Autodesk Inventor part; units mm, degrees
ref_plane "YZ Plane" through (0, 0, 0) normal (1, 0, 0) x (0, 1, 0)
ref_plane "XZ Plane" through (0, 0, 0) normal (0, 1, 0) x (-1, 0, 0)
ref_plane "XY Plane" through (0, 0, 0) normal (0, 0, 1) x (1, 0, 0)
sketch "Sketch1" plane through (0, 0, 0) normal (0, 1, 0) x (-1, 0, 0)
  line L0 (65, 0) -> (65, -110)
  line L1 (65, -110) -> (0, -110)
  line L2 (0, -110) -> (0, 0)
  line L3 (65, 0) -> (65, -34.9842)
  line L4 (65, 0) -> (50.25, 0)
  line L5 (50.25, 0) -> (50.25, -30.5)
  line L6 (0, 0) -> (14.75, 0)
  line L7 (14.75, 0) -> (14.75, -30.5)
  line L8 (50.25, -30.5) -> (14.75, -30.5)
  line L9 (0, 0) -> (14.75, 0)
  line L10 (50.25, 0) -> (65, 0)
  dimension "d0" = 65
  dimension "d1" = 110
  dimension "d2" = 14.75
  dimension "d3" = 30.5
  dimension "d4" = 14.75
  dimension "d5" = 30.5
extrude "Extrusion1" add sketch "Sketch1" along normal blind 18.5
sketch "Sketch2" plane through (0, 18.5, 0) normal (0, 1, 0) x (1, 0, 0)
  line L0 (0, 110) -> (-65, 110)
  line L1 (-65, 110) -> (-65, 0)
  line L2 (-14.75, 0) -> (0, 0)
  line L3 (-65, 0) -> (0, 0)
  line L4 (0, 0) -> (0, 110)
  line L5 (-65, 110) -> (-65, 0)
  line L6 (0, 110) -> (-65, 110)
extrude "Extrusion2" add sketch "Sketch2" along normal blind 10
sketch "Sketch3" plane through (0, 0, 0) normal (0, -1, 0) x (1, 0, 0)
  line L0 (0, 0) -> (0, -110)
  line L1 (0, -110) -> (-65, -110)
  line L2 (0, 0) -> (0, -110)
  line L3 (0, -110) -> (-65, -110)
  line L4 (-65, -110) -> (-65, 0)
  line L5 (-65, -110) -> (-65, 0)
  line L6 (-65, 0) -> (0, 0)
extrude "Extrusion3" add sketch "Sketch3" along normal blind 10
sketch "Sketch4" plane through (0, -10, 0) normal (0, -1, 0) x (1, 0, 0)
  line L0 (0, 0) -> (0, -110)
  line L1 (0, -110) -> (0, -102)
  line L2 (0, -110) -> (-32.5, -110)
  line L3 (-32.5, -110) -> (-24.5, -110)
  line L4 (0, -110) -> (-65, -110)
  line L5 (-32.5, -110) -> (-32.5, -102)
  line L6 (-32.5, -102) -> (-11.25, -102)
  line L7 (-11.25, -102) -> (-11.25, -91.5)
  line L8 (-11.25, -91.5) -> (-53.75, -91.5)
  line L9 (-53.75, -91.5) -> (-53.75, -102)
  line L10 (-53.75, -102) -> (-32.5, -102)
  dimension "d19" = 32.5
  dimension "d26" = 8
  dimension "d27" = 21.25
  dimension "d28" = 10.5
  dimension "d29" = 42.5
  dimension "d30" = 10.5
extrude "Extrusion4" cut sketch "Sketch4" against normal through all
properties part number "techo2"
Geometry check sheet. Reference: the model listing, model coordinates, mm. A direction names the side the tool comes from. Coordinates: 2 decimals unless noted, no trailing zeros. Loops run counter-clockwise (first coordinate to the right, second up) from the corner with the lowest first, then second, coordinate; pieces in that order, holes last. Notation, with made-up numbers: (42.25, 58) - (67.25, 58) arc R19 ccw to (67.25, 95) - close; hole circle Ø11 at (11, 85.5). An arc over 180 degrees is marked (long way). One line per item, written item: value. Start each with the question number.
(1) Material ranges on line 1 (X direction, y = 3.5, z = -25); line 2 (Z direction, x = -46, y = 16); line 3 (Z direction, x = -53.5, y = -3.5), recorded low to high. Write a range as [from, to].
(2) Depth check by flat-ended pin: P1, Ø4, axis at x = -36, y = 8.5, coming from the +Z side. Enter the tip coordinate at first touch or a pass-through.
(3) Mould release check, pull along Z, two halves, no side actions. Record for faces 4 (the flat face through (-33, 0, -15)), 5 (the flat face through (-33, 22, 0)), 6 (the flat face through (-32, 9, -91.5)): released by +Z, released by -Z, zero draft, split by the parting line, or undercut.
(4) Cross-section at A-A on x = -40. Enter the section's corners in (y, z), plus the area to 3 significant figures.
(5) Cross-section at C-C on y = 26. Enter the section's corners in (x, z), plus the area to 3 significant figures.
(6) Cross-section at B-B on z = -27.5. Enter the section's corners in (x, y), plus the area to 3 significant figures.
(7) Tool access check on faces 1 (the flat face through (-11.25, 9, -97)), 2 (the flat face through (-33, 18.5, -15)), 3 (the flat face through (-65, 10, -56)). Record the directions out of +Z, -Z, +X, -X, +Y, -Y that give a thin tool (end or side, any length) a straight path to the whole face; none if there is none.
(8) Cross-section at D-D on y = 4. Enter the section's corners in (x, z), plus the area to 3 significant figures.
Results below:
1. line 1: x = [-65, -50.25], [-14.75, 0]
1. line 2: z = [-110, -102], [-91.5, -30.5]
1. line 3: z = [-110, -102], [-91.5, 0]
2. P1: stops at z = -30.5
3. face 4: zero draft
3. face 5: released by +Z
3. face 6: undercut
4. outline: (-10, -110) - (28.5, -110) - (28.5, -102) - (-10, -102) - close; (-10, -91.5) - (28.5, -91.5) - (28.5, 0) - (18.5, 0) - (18.5, -30.5) - (0, -30.5) - (0, 0) - (-10, 0) - close
4. area: 3,270 mm2
5. outline: (-65, -110) - (0, -110) - (0, 0) - (-65, 0) - close; hole (-53.75, -102) - (-11.25, -102) - (-11.25, -91.5) - (-53.75, -91.5) - close
5. area: 6,700 mm2
6. outline: (-65, -10) - (0, -10) - (0, 28.5) - (-65, 28.5) - close; hole (-50.25, 0) - (-14.75, 0) - (-14.75, 18.5) - (-50.25, 18.5) - close
6. area: 1,850 mm2
7. face 1: +Y, -Y
7. face 2: +Z
7. face 3: +Z, -Z, -X, +Y, -Y
8. outline: (-65, -110) - (0, -110) - (0, 0) - (-14.75, 0) - (-14.75, -30.5) - (-50.25, -30.5) - (-50.25, 0) - (-65, 0) - close; hole (-53.75, -102) - (-11.25, -102) - (-11.25, -91.5) - (-53.75, -91.5) - close
8. area: 5,620 mm2
